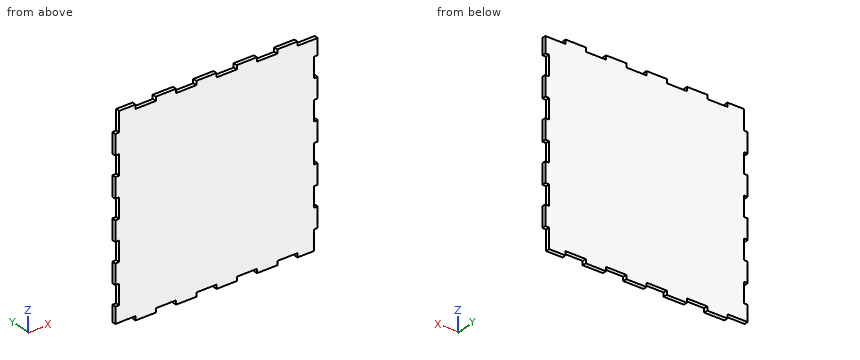
from build123d import *

# Parameters (mm, degrees)
F1_DEPTH = 5.5


with BuildPart() as f1:
    # F0 (on Front) → F1 (new body)
    with BuildSketch(Plane.XZ):
        Polygon((-114, 137.5), (-137, 137.5), (-137, 110), (-142.5, 110), (-142.5, 82.5), (-137, 82.5), (-137, 55), (-142.5, 55), (-142.5, 27.5), (-137, 27.5), (-137, 0), (-142.5, 0), (-142.5, -27.5), (-137, -27.5), (-137, -55), (-142.5, -55), (-142.5, -82.5), (-137, -82.5), (-137, -110), (-142.5, -110), (-142.5, -132), (-114, -132), (-114, -137.5), (-85.5, -137.5), (-85.5, -132), (-57, -132), (-57, -137.5), (-28.5, -137.5), (-28.5, -132), (0, -132), (0, -137.5), (28.5, -137.5), (28.5, -132), (57, -132), (57, -137.5), (85.5, -137.5), (85.5, -132), (114, -132), (114, -137.5), (137, -137.5), (137, -110), (142.5, -110), (142.5, -82.5), (137, -82.5), (137, -55), (142.5, -55), (142.5, -27.5), (137, -27.5), (137, 0), (142.5, 0), (142.5, 27.5), (137, 27.5), (137, 55), (142.5, 55), (142.5, 82.5), (137, 82.5), (137, 110), (142.5, 110), (142.5, 132), (114, 132), (114, 137.5), (85.5, 137.5), (85.5, 132), (57, 132), (57, 137.5), (28.5, 137.5), (28.5, 132), (0, 132), (0, 137.5), (-28.5, 137.5), (-28.5, 132), (-57, 132), (-57, 137.5), (-85.5, 137.5), (-85.5, 132), (-114, 132), align=None)
    extrude(amount=F1_DEPTH)


solid = f1.part
CAD build for the part. Positions are in the model's coordinates, mm. Coordinates: 2 decimals unless noted, no trailing zeros. Loops run counter-clockwise (first coordinate to the right, second up) from the corner with the lowest first, then second, coordinate; pieces in that order, holes last. Notation, with made-up numbers: (24.5, 9.25) - (48.5, 9.25) arc R16 cw to (48.5, 30.25) - close; hole circle Ø7 at (-18.75, -15). An arc over 180 degrees is marked (long way). Write item = value, one per line. Start each with the question number.
Q1. Cut at B-B, the plane x = 73. List the corners of the cut face in (y, z).
Q2. Cut at A-A, the plane z = -37. List the corners of the cut face in (x, y), then the cut area to 3 significant figures.
Q3. Drill centre lines: L1, parallel to X at y = -1.1, z = 20; L2, parallel to X at y = -0.2, z = 99.5; L3, parallel to Z at x = 26, y = -3.45. Where is each one in solid material? Low to high.
Q4. Flat gauge pins, fed straight in: pin 1 Ø3 at (x, y) = (-139, -3) entering from +Z; pin 2 Ø1.5 at (y, z) = (-3, -60) entering from +X; pin 3 Ø1.6 at (y, z) = (-3, -135) entering from -X. Where does each tip first touch, or does it go through?
Computed:
q1.outline = (-5.5, -137.5) - (0, -137.5) - (0, 132) - (-5.5, 132) - close
q2.outline = (-137, -5.5) - (142.5, -5.5) - (142.5, 0) - (-137, 0) - close
q2.area = 1,540 mm²
q3.L1 = -137 to 142.5
q3.L2 = -142.5 to 137
q3.L3 = -137.5 to 132
q4.pin_1 = 110
q4.pin_2 = 137
q4.pin_3 = -114
